Work out the finished part from the listing and answer in its coordinate system (mm). A direction names the side the tool comes from. Round coordinates to 2 decimals unless told otherwise and drop trailing zeros. Order: outer loops, then holes, each group sorted by start corner. A loop starts at its lowest first (then second) coordinate and runs counter-clockwise, first axis right, second up. Notation, with made-up numbers: (6.5, 42.25) - (32.5, 42.25) arc R33 ccw to (32.5, 72.25) - close; hole circle Ø3 at (63, 37.5). An arc over 180 degrees is marked (long way). Use one line per item in the form item = value. Start each with the question number.
Q1. Find the intervals of material crossed by line 1 (Y direction, x = -4.5, z = 1.85); line 2 (Y direction, x = -4.25, z = 2.05); line 3 (Z direction, x = 2, y = 29.5), in increasing order. Write a range as [from, to].
Q2. Given P1, Ø2.5, axis at x = -0.5, y = 0.5, coming from the +Z side; P2, Ø4, axis at x = -2, y = 20.5, coming from the +Z side; P3, Ø4, axis at x = -1, y = 30.5, coming from the +Z side, each flat-ended and moving along its own axis, determine where each tip first touches the part or whether it passes through.
Q3. The part is cut by section C-C on z = 1.5. Determine the outline of the cut face in (x, y), plus the area to 3 significant figures.
Q4. The part is cut by section A-A on x = 2.25. Determine the outline of the cut face in (y, z), plus the area to 4 significant figures.
Q5. The part is cut by section B-B on y = 26. Determine the outline of the cut face in (x, z).
Q6. Which of the six approach directions +Z, -Z, +X, -X, +Y, -Y give full straight-line access (tool end or side, diameter ignored) to faces 1 (the flat face through (-1, -10, 4.3)), 2 (the flat face through (-1, 20, 2.6))?
from build123d import *

# Parameters (mm, degrees)
F0_W      = 5
F0_H      = 5
F1_DEPTH  = 1
F2_DEPTH  = 2
F3_DEPTH  = 2.3
F4_DEPTH  = 2.6
F5_DEPTH  = 2.9
F6_DEPTH  = 3.1
F7_DEPTH  = 3.4
F8_DEPTH  = 3.7
F9_DEPTH  = 4
F10_DEPTH = 4.3


with BuildPart() as f1:
    # F0 (on Top) → F1 (new body)
    with BuildSketch(Plane.XY):
        with Locations((-3.713795, 34.692926)):
            Rectangle(F0_W, F0_H)
        with Locations((1.286205, 34.692926)):
            Rectangle(F0_W, F0_H)
    extrude(amount=F1_DEPTH)

    # F0 (on Top) → F2 (join)
    with BuildSketch(Plane.XY):
        with Locations((-3.713795, 29.692926)):
            Rectangle(F0_W, F0_H)
        with Locations((1.286205, 29.692926)):
            Rectangle(F0_W, F0_H)
    extrude(amount=F2_DEPTH)

    # F0 (on Top) → F3 (join)
    with BuildSketch(Plane.XY):
        with Locations((-3.713795, 24.692926)):
            Rectangle(F0_W, F0_H)
        with Locations((1.286205, 24.692926)):
            Rectangle(F0_W, F0_H)
    extrude(amount=F3_DEPTH)

    # F0 (on Top) → F4 (join)
    with BuildSketch(Plane.XY):
        with Locations((1.286205, 19.692926)):
            Rectangle(F0_W, F0_H)
        with Locations((-3.713795, 19.692926)):
            Rectangle(F0_W, F0_H)
    extrude(amount=F4_DEPTH)

    # F0 (on Top) → F5 (join)
    with BuildSketch(Plane.XY):
        with Locations((-3.713795, 14.692926)):
            Rectangle(F0_W, F0_H)
        with Locations((1.286205, 14.692926)):
            Rectangle(F0_W, F0_H)
    extrude(amount=F5_DEPTH)

    # F0 (on Top) → F6 (join)
    with BuildSketch(Plane.XY):
        with Locations((-3.713795, 9.692926)):
            Rectangle(F0_W, F0_H)
        with Locations((1.286205, 9.692926)):
            Rectangle(F0_W, F0_H)
    extrude(amount=F6_DEPTH)

    # F0 (on Top) → F7 (join)
    with BuildSketch(Plane.XY):
        with Locations((-3.713795, 4.692926)):
            Rectangle(F0_W, F0_H)
        with Locations((1.286205, 4.692926)):
            Rectangle(F0_W, F0_H)
    extrude(amount=F7_DEPTH)

    # F0 (on Top) → F8 (join)
    with BuildSketch(Plane.XY):
        with Locations((-3.713795, -0.307074)):
            Rectangle(F0_W, F0_H)
        with Locations((1.286205, -0.307074)):
            Rectangle(F0_W, F0_H)
    extrude(amount=F8_DEPTH)

    # F0 (on Top) → F9 (join)
    with BuildSketch(Plane.XY):
        with Locations((-3.713795, -5.307074)):
            Rectangle(F0_W, F0_H)
        with Locations((1.286205, -5.307074)):
            Rectangle(F0_W, F0_H)
    extrude(amount=F9_DEPTH)

    # F0 (on Top) → F10 (join)
    with BuildSketch(Plane.XY):
        with Locations((-3.713795, -10.307074)):
            Rectangle(F0_W, F0_H)
        with Locations((1.286205, -10.307074)):
            Rectangle(F0_W, F0_H)
    extrude(amount=F10_DEPTH)


solid = f1.part
Found:
q1.line_1 = [-12.81, 32.19]
q1.line_2 = [-12.81, 27.19]
q1.line_3 = [0, 2]
q2.P1 = 3.7
q2.P2 = 2.6
q2.P3 = 2
q3.outline = (-6.21, -12.81) - (3.79, -12.81) - (3.79, 32.19) - (-6.21, 32.19) - close
q3.area = 450 mm²
q4.outline = (-12.81, 0) - (37.19, 0) - (37.19, 1) - (32.19, 1) - (32.19, 2) - (27.19, 2) - (27.19, 2.3) - (22.19, 2.3) - (22.19, 2.6) - (17.19, 2.6) - (17.19, 2.9) - (12.19, 2.9) - (12.19, 3.1) - (7.19, 3.1) - (7.19, 3.4) - (2.19, 3.4) - (2.19, 3.7) - (-2.81, 3.7) - (-2.81, 4) - (-7.81, 4) - (-7.81, 4.3) - (-12.81, 4.3) - close
q4.area = 146.5 mm²
q5.outline = (-6.21, 0) - (3.79, 0) - (3.79, 2.3) - (-6.21, 2.3) - close
q6.face_1 = +Z, +X, -X, +Y, -Y
q6.face_2 = +Z, +X, -X, +Y
